from build123d import *

# Parameters (mm, degrees)
SKETCH1_W                  = 45
SKETCH1_H                  = 45
BOSS_EXTRUDE1_DEPTH        = 30
BOSS_EXTRUDE1_DEPTH_BACK   = 35
F_22_0_22_DIAMETER_HOLE1_D = 22
F_22_0_22_DIAMETER_HOLE2_D = 22
SKETCH7_R                  = 12.8397
CUT_EXTRUDE1_DEPTH         = 9
CUT_EXTRUDE2_DEPTH         = 13.2
CUT_EXTRUDE3_REACH         = 29.667
SKETCH9_W                  = 26.4
SKETCH9_H                  = 36
FILLET1_R                  = 2
CUT_EXTRUDE6_REACH         = 29.667
CUT_EXTRUDE4_DEPTH         = 4.499464
CUT_EXTRUDE5_DEPTH         = 9.772078
CUT_EXTRUDE7_DEPTH         = 15
BOSS_EXTRUDE2_DEPTH        = 1.5
M2_TAPPED_HOLE1_D          = 1.6
M2_TAPPED_HOLE1_DEPTH      = 3.2
M2_TAPPED_HOLE1_TIP        = 0.480688495
M2_TAPPED_HOLE2_D          = 1.6
M2_TAPPED_HOLE2_DEPTH      = 5.2
M2_TAPPED_HOLE2_TIP        = 0.480688495
M2_TAPPED_HOLE3_D          = 1.6
M2_TAPPED_HOLE3_DEPTH      = 5.2
M2_TAPPED_HOLE3_TIP        = 0.480688495
M3_TAPPED_HOLE1_D          = 2.5
M3_TAPPED_HOLE2_D          = 2.5
M3_TAPPED_HOLE2_DEPTH      = 7.5
M3_TAPPED_HOLE2_TIP        = 0.751075774
M2_TAPPED_HOLE4_D          = 1.6
M2_TAPPED_HOLE4_DEPTH      = 5.2
M2_TAPPED_HOLE4_TIP        = 0.480688495
CUT_EXTRUDE8_REACH         = 47
SKETCH30_R                 = 8.75
F_4_40_TAPPED_HOLE1_D      = 2.2606
F_4_40_TAPPED_HOLE1_DEPTH  = 4.2
F_4_40_TAPPED_HOLE1_TIP    = 0.679152758
F_4_40_TAPPED_HOLE2_D      = 2.2606
F_4_40_TAPPED_HOLE2_DEPTH  = 5.18
F_4_40_TAPPED_HOLE2_TIP    = 0.679152758


with BuildPart() as part:
    # Sketch1 → Boss-Extrude1 (new body, two sides)
    with BuildSketch(Plane(origin=(0, 0, 0), x_dir=(1, 0, 0), z_dir=(0, 1, 0))) as boss_extrude1_sk:
        Rectangle(SKETCH1_W, SKETCH1_H)
    extrude(amount=BOSS_EXTRUDE1_DEPTH)
    extrude(boss_extrude1_sk.sketch, amount=-BOSS_EXTRUDE1_DEPTH_BACK)

    # Ø22.0 (22) Diameter Hole1 (through all)
    with Locations(Plane(origin=(0, 30, 0), x_dir=(1, 0, 0), z_dir=(0, 1, 0))):
        with Locations((0, 0)):
            Hole(F_22_0_22_DIAMETER_HOLE1_D / 2)

    # Ø22.0 (22) Diameter Hole2 (through all)
    with Locations(Plane.XY.offset(22.5)):
        with Locations((0, -17.5)):
            Hole(F_22_0_22_DIAMETER_HOLE2_D / 2)

    # Sketch7 → Cut-Extrude1 (cut)
    with BuildSketch(Plane.XY.offset(22.5)):
        with Locations((0, -17.5)):
            Circle(SKETCH7_R)
    extrude(amount=-CUT_EXTRUDE1_DEPTH, mode=Mode.SUBTRACT)

    # Sketch8 → Cut-Extrude2 (cut, symmetric)
    with BuildSketch(Plane.XY):
        Polygon((-12.727922061, 2.272077939), (-11.914749263, 1.45890514), (13.54109486, 26.914749263), (12.727922061, 27.727922061), align=None)
    extrude(amount=CUT_EXTRUDE2_DEPTH, both=True, mode=Mode.SUBTRACT)

    # Sketch9 → Cut-Extrude3 (cut, up to next)
    with BuildSketch(Plane(origin=(-6.686827202, 6.686827202, 0), x_dir=(0, 0, 1), z_dir=(-0.707106781, 0.707106781, 0)), mode=Mode.PRIVATE) as cut_extrude3_sk1:
        with Locations((0, 10.606601718)):
            Rectangle(SKETCH9_W, SKETCH9_H)
    cut_extrude3_tool1 = extrude(cut_extrude3_sk1.sketch, amount=CUT_EXTRUDE3_REACH, mode=Mode.PRIVATE) & part.part
    add(cut_extrude3_tool1.solids().sort_by_distance((0.813173, 14.186827, 0))[0], mode=Mode.SUBTRACT)

    # Fillet1
    fillet1_edges = [part.edges().sort_by_distance(p)[0] for p in [
        (11.998469491, 28.457374631, -13.2),
        (-17.207374631, 6.751530509, -13.2),
        (-17.207374631, 6.751530509, 13.2),
        (11.998469491, 28.457374631, 13.2),
    ]]
    fillet(fillet1_edges, radius=FILLET1_R)

    # Sketch12 → Cut-Extrude6 (cut, up to next)
    with BuildSketch(Plane(origin=(-6.686827202, 6.686827202, 0), x_dir=(0, 0, 1), z_dir=(-0.707106781, 0.707106781, 0)), mode=Mode.PRIVATE) as cut_extrude6_sk1:
        with BuildLine():
            Line((-9.2, -5.393398282), (-9.2, -7.393398282))
            ThreePointArc((-9.2, -7.393398282), (-11.2, -9.393398282), (-13.2, -7.393398282))
            Line((-13.2, -7.393398282), (-13.2, -5.393398282))
            ThreePointArc((-13.2, -5.393398282), (-11.2, -3.393398282), (-9.2, -5.393398282))
        make_face()
    cut_extrude6_tool1 = extrude(cut_extrude6_sk1.sketch, amount=CUT_EXTRUDE6_REACH, mode=Mode.PRIVATE) & part.part
    add(cut_extrude6_tool1.solids().sort_by_distance((-11.207642, 2.166012, -11.2))[0], mode=Mode.SUBTRACT)
    # Sketch12 → Cut-Extrude6 (cut, up to next)
    with BuildSketch(Plane(origin=(-6.686827202, 6.686827202, 0), x_dir=(0, 0, 1), z_dir=(-0.707106781, 0.707106781, 0)), mode=Mode.PRIVATE) as cut_extrude6_sk2:
        with BuildLine():
            Line((13.2, -5.393398282), (13.2, -7.393398282))
            ThreePointArc((13.2, -7.393398282), (11.2, -9.393398282), (9.2, -7.393398282))
            Line((9.2, -7.393398282), (9.2, -5.393398282))
            ThreePointArc((9.2, -5.393398282), (11.2, -3.393398282), (13.2, -5.393398282))
        make_face()
    cut_extrude6_tool2 = extrude(cut_extrude6_sk2.sketch, amount=CUT_EXTRUDE6_REACH, mode=Mode.PRIVATE) & part.part
    add(cut_extrude6_tool2.solids().sort_by_distance((-11.207642, 2.166012, 11.2))[0], mode=Mode.SUBTRACT)

    # Sketch10 → Cut-Extrude4 (cut)
    with BuildSketch(Plane(origin=(0, 30, 0), x_dir=(1, 0, 0), z_dir=(0, 1, 0))):
        with BuildLine():
            Line((7.627416998, 13.2), (15.5, 13.2))
            ThreePointArc((15.5, 13.2), (16.914213562, 12.614213562), (17.5, 11.2))
            Line((17.5, 11.2), (17.5, -11.2))
            ThreePointArc((17.5, -11.2), (16.914213562, -12.614213562), (15.5, -13.2))
            Line((15.5, -13.2), (7.627416998, -13.2))
            Line((7.627416998, -13.2), (7.627416998, 13.2))
        make_face()
    extrude(amount=-CUT_EXTRUDE4_DEPTH, mode=Mode.SUBTRACT)

    # Sketch11 → Cut-Extrude5 (cut)
    with BuildSketch(Plane.ZY.offset(22.5)):
        with BuildLine():
            Line((-18.2, 30), (18.2, 30))
            Line((18.2, 30), (18.2, 4.272077939))
            ThreePointArc((18.2, 4.272077939), (17.614213562, 2.857864376), (16.2, 2.272077939))
            Line((16.2, 2.272077939), (-16.2, 2.272077939))
            ThreePointArc((-16.2, 2.272077939), (-17.614213562, 2.857864376), (-18.2, 4.272077939))
            Line((-18.2, 4.272077939), (-18.2, 30))
        make_face()
    extrude(amount=-CUT_EXTRUDE5_DEPTH, mode=Mode.SUBTRACT)

    # Sketch13 → Cut-Extrude7 (cut, symmetric)
    with BuildSketch(Plane(origin=(0, 0, 0), x_dir=(0, 0, -1), z_dir=(1, 0, 0))):
        Polygon((-17.5, -35), (22.5, 5), (22.5, -35), align=None)
    extrude(amount=CUT_EXTRUDE7_DEPTH, both=True, mode=Mode.SUBTRACT)

    # Sketch18 → Boss-Extrude2 (add)
    with BuildSketch(Plane(origin=(0, 30, 0), x_dir=(1, 0, 0), z_dir=(0, 1, 0))):
        with BuildLine():
            Line((-12.727922061, -13.2), (-12.727922061, -18.2))
            Line((-12.727922061, -18.2), (-22.5, -18.2))
            Line((-22.5, -18.2), (-22.5, -22.5))
            Line((-22.5, -22.5), (22.5, -22.5))
            Line((22.5, -22.5), (22.5, 22.5))
            Line((22.5, 22.5), (-22.5, 22.5))
            Line((-22.5, 22.5), (-22.5, 18.2))
            Line((-22.5, 18.2), (-12.727922061, 18.2))
            Line((-12.727922061, 18.2), (-12.727922061, 13.2))
            Line((-12.727922061, 13.2), (15.5, 13.2))
            ThreePointArc((15.5, 13.2), (16.914213562, 12.614213562), (17.5, 11.2))
            Line((17.5, 11.2), (17.5, -11.2))
            ThreePointArc((17.5, -11.2), (16.914213562, -12.614213562), (15.5, -13.2))
            Line((15.5, -13.2), (-12.727922061, -13.2))
        make_face()
    extrude(amount=BOSS_EXTRUDE2_DEPTH)

    # M2 Tapped Hole1
    with Locations(Plane(origin=(0, -8.75, -8.75), x_dir=(-1, 0, 0), z_dir=(0, -0.707106781, -0.707106781))):
        with Locations((11.75, -28.123106012), (11.75, 10.876893988), (-11.75, 10.876893988), (-11.75, -28.123106012)):
            Hole(M2_TAPPED_HOLE1_D / 2, depth=M2_TAPPED_HOLE1_DEPTH)
            with Locations((0, 0, -(M2_TAPPED_HOLE1_DEPTH + M2_TAPPED_HOLE1_TIP / 2))):  # 118° drill point
                Cone(0, M2_TAPPED_HOLE1_D / 2, M2_TAPPED_HOLE1_TIP, mode=Mode.SUBTRACT)

    # M2 Tapped Hole2
    with Locations(Plane(origin=(0, 25.500535701, 0), x_dir=(1, 0, 0), z_dir=(0, 1, 0))):
        with Locations((14.5, 7), (14.5, -7)):
            Hole(M2_TAPPED_HOLE2_D / 2, depth=M2_TAPPED_HOLE2_DEPTH)
            with Locations((0, 0, -(M2_TAPPED_HOLE2_DEPTH + M2_TAPPED_HOLE2_TIP / 2))):  # 118° drill point
                Cone(0, M2_TAPPED_HOLE2_D / 2, M2_TAPPED_HOLE2_TIP, mode=Mode.SUBTRACT)

    # M2 Tapped Hole3
    with Locations(Plane(origin=(0, 31.5, 0), x_dir=(1, 0, 0), z_dir=(0, 1, 0))):
        with Locations((-5, 18.5), (18.5, 18.5), (-5, -18.5), (18.5, -18.5)):
            Hole(M2_TAPPED_HOLE3_D / 2, depth=M2_TAPPED_HOLE3_DEPTH)
            with Locations((0, 0, -(M2_TAPPED_HOLE3_DEPTH + M2_TAPPED_HOLE3_TIP / 2))):  # 118° drill point
                Cone(0, M2_TAPPED_HOLE3_D / 2, M2_TAPPED_HOLE3_TIP, mode=Mode.SUBTRACT)

    # M3 Tapped Hole1 (through all)
    with Locations(Plane.ZY.offset(22.5)):
        with Locations((-10, -31), (10, -31)):
            Hole(M3_TAPPED_HOLE1_D / 2)

    # M3 Tapped Hole2
    with Locations(Plane(origin=(0, -35, 0), x_dir=(-1, 0, 0), z_dir=(0, -1, 0))):
        with Locations((-19, -19), (19, 19), (19, -19), (-19, 19)):
            Hole(M3_TAPPED_HOLE2_D / 2, depth=M3_TAPPED_HOLE2_DEPTH)
            with Locations((0, 0, -(M3_TAPPED_HOLE2_DEPTH + M3_TAPPED_HOLE2_TIP / 2))):  # 118° drill point
                Cone(0, M3_TAPPED_HOLE2_D / 2, M3_TAPPED_HOLE2_TIP, mode=Mode.SUBTRACT)

    # M2 Tapped Hole4
    with Locations(Plane.ZY.offset(12.727922061)):
        with Locations((-14.7, 24), (14.7, 24)):
            Hole(M2_TAPPED_HOLE4_D / 2, depth=M2_TAPPED_HOLE4_DEPTH)
            with Locations((0, 0, -(M2_TAPPED_HOLE4_DEPTH + M2_TAPPED_HOLE4_TIP / 2))):  # 118° drill point
                Cone(0, M2_TAPPED_HOLE4_D / 2, M2_TAPPED_HOLE4_TIP, mode=Mode.SUBTRACT)

    # Sketch30 → Cut-Extrude8 (cut, up to next)
    with BuildSketch(Plane(origin=(22.5, 0, 0), x_dir=(0, 0, -1), z_dir=(1, 0, 0)), mode=Mode.PRIVATE) as cut_extrude8_sk1:
        with Locations((0, 13.373654403)):
            Circle(SKETCH30_R)
    cut_extrude8_tool1 = extrude(cut_extrude8_sk1.sketch, amount=-CUT_EXTRUDE8_REACH, mode=Mode.PRIVATE) & part.part
    add(cut_extrude8_tool1.solids().sort_by_distance((22.5, 13.373654, 0))[0], mode=Mode.SUBTRACT)

    # #4-40 Tapped Hole1
    with Locations(Plane(origin=(22.5, 0, 0), x_dir=(0, 0, -1), z_dir=(1, 0, 0))):
        with Locations((-15, 28.373654403), (-15, -1.626345597), (15, -1.626345597), (15, 28.373654403)):
            Hole(F_4_40_TAPPED_HOLE1_D / 2, depth=F_4_40_TAPPED_HOLE1_DEPTH)
            with Locations((0, 0, -(F_4_40_TAPPED_HOLE1_DEPTH + F_4_40_TAPPED_HOLE1_TIP / 2))):  # 118° drill point
                Cone(0, F_4_40_TAPPED_HOLE1_D / 2, F_4_40_TAPPED_HOLE1_TIP, mode=Mode.SUBTRACT)

    # #4-40 Tapped Hole2
    with Locations(Plane.XY.offset(22.5)):
        with Locations((-15, -2.5), (15, -2.5), (-15, -32.5), (15, -32.5)):
            Hole(F_4_40_TAPPED_HOLE2_D / 2, depth=F_4_40_TAPPED_HOLE2_DEPTH)
            with Locations((0, 0, -(F_4_40_TAPPED_HOLE2_DEPTH + F_4_40_TAPPED_HOLE2_TIP / 2))):  # 118° drill point
                Cone(0, F_4_40_TAPPED_HOLE2_D / 2, F_4_40_TAPPED_HOLE2_TIP, mode=Mode.SUBTRACT)


solid = part.part
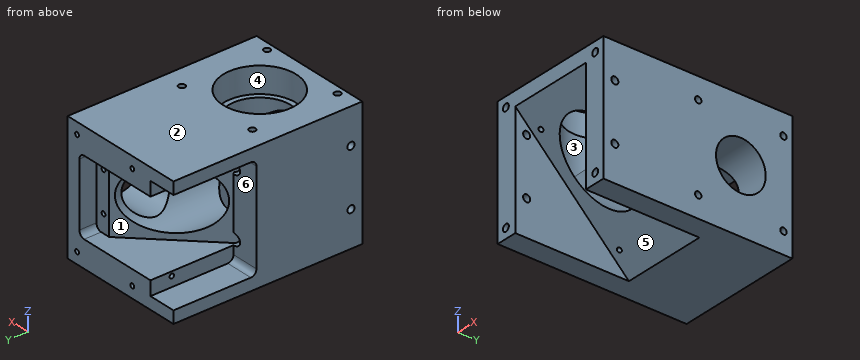
Build history of the part. All positions in model axes, mm. Face numbers are marked on the shaded views. A direction names the side the tool comes from. Coordinates: 2 decimals unless noted, no trailing zeros. Order: outer loops, then holes, each group sorted by start corner. A loop starts at its lowest first (then second) coordinate and runs counter-clockwise, first axis right, second up. Notation, with made-up numbers: (31, 18) - (57, 18) arc R4 cw to (57, 24) - close; hole circle Ø1 at (11.5, 44.5). An arc over 180 degrees is marked (long way). Write item = value, one per line. Start each with the question number.
1) Saw through at A-A on z = -1. Write the cut outline in (x, y), then the cut area to 3 significant figures.
2) Flat gauge pins, fed straight in: pin 1 Ø1.3 at (x, z) = (14.5, 7) entering from +Y; pin 2 Ø1.4 at (y, z) = (24, -14.7) entering from -X; pin 3 Ø2 at (x, z) = (19, 19) entering from -Y; pin 4 Ø1 at (x, z) = (-5, -8.5) entering from -Y. Where does each tip first touch, or does it go through?
3) 3-axis set-ups, long thin cutter, end or side, ignore diameter. For the marked faces 4, 5 and 6: which of +Z, -Z, +X, -X, +Y, -Y reach the whole face in a straight line?
4) Two-plate mould, pull along Y, no slides. Class the marked faces 1, 2 and 3: pulls with the +Y half, pulls with the -Y half, needs draft (parallel to the pull), parting line crosses it, or undercut.
5) Saw through at D-D on z = -10. Write the cut outline in (x, y).
6) Wall check: line 1 along X through (y, z) = (29.3, -18.5); line 2 along Z through (x, y) = (-5, 27); line 3 along Y through (x, z) = (21.15, -15). Give the ranges that are in metal, low to high. Write a range as from..to.
7) Saw through at B-B on x = 3.5. Write the cut outline in (y, z).
8) Saw through at C-C on y = 17. Write the cut outline in (x, z), then the cut area to 3 significant figures.
From the geometry:
q1.outline = (-22.5, -35) - (-15, -35) - (-15, -16.5) - (-10.95, -16.5) - (-10.95, 2.42) - (-11.91, 1.46) - (-12.73, 2.27) - (-22.5, 2.27) - close; (10.95, -16.5) - (15, -16.5) - (15, -35) - (22.5, -35) - (22.5, 4.68) - (10.95, 4.68) - close; (10.95, 22.07) - (22.5, 22.07) - (22.5, 31.5) - (17.5, 31.5) - (17.5, 25.5) - (12.13, 25.5) - (10.95, 24.33) - close
q1.area = 807 mm^2
q2.pin_1 = 20.21
q2.pin_2 = -7.47
q2.pin_3 = -27.35
q2.pin_4 = through
q3.face_4 = +Z
q3.face_5 = -Z, -Y
q3.face_6 = -X, +Y
q4.face_1 = pulls with the +Y half
q4.face_2 = needs draft
q4.face_3 = undercut
q5.outline = (-22.5, -35) - (-15, -35) - (-15, -32.25) - (-22.5, -32.25) - close; (-22.5, -29.75) - (-15, -29.75) - (-15, -7.5) - (-4.58, -7.5) - (-4.58, 8.79) - (-13.05, 0.33) - (-14.99, 2.27) - (-22.5, 2.27) - close; (4.58, -7.5) - (15, -7.5) - (15, -29.75) - (22.5, -29.75) - (22.5, 31.5) - (17.5, 31.5) - (17.5, 25.5) - (12.13, 25.5) - (4.58, 17.96) - close; (15, -35) - (22.5, -35) - (22.5, -32.25) - (15, -32.25) - close
q6.line_1 = -22.5..-5.8, -4.2..17.7, 19.3..22.5
q6.line_2 = -22.5..-19.3, -17.7..-13.2, 13.2..17.7, 19.3..22.5
q6.line_3 = -35..-2.76, -0.5..27.24, 29.5..31.5
q7.outline = (-35, 17.5) - (-27.93, 10.43) - (-27.93, 13.5) - (-29.85, 13.5) - (-29.85, 22.5) - (-35, 22.5) - close; (-7.07, -10.43) - (5, -22.5) - (31.5, -22.5) - (31.5, -13.2) - (16.87, -13.2) - (16.87, -10.43) - close; (-7.07, 10.43) - (16.87, 10.43) - (16.87, 13.2) - (31.5, 13.2) - (31.5, 22.5) - (-5.15, 22.5) - (-5.15, 13.5) - (-7.07, 13.5) - close
q8.outline = (-22.5, -22.5) - (22.5, -22.5) - (22.5, -7.96) - (7.59, -7.96) arc R11 cw to (3.63, -10.39) - (3.63, -13.2) - (-12.73, -13.2) - (-12.73, -18.2) - (-22.5, -18.2) - close; (-22.5, 18.2) - (-12.73, 18.2) - (-12.73, 13.2) - (3.63, 13.2) - (3.63, 10.39) arc R11 cw to (7.59, 7.96) - (22.5, 7.96) - (22.5, 22.5) - (-22.5, 22.5) - close
q8.area = 926 mm^2
